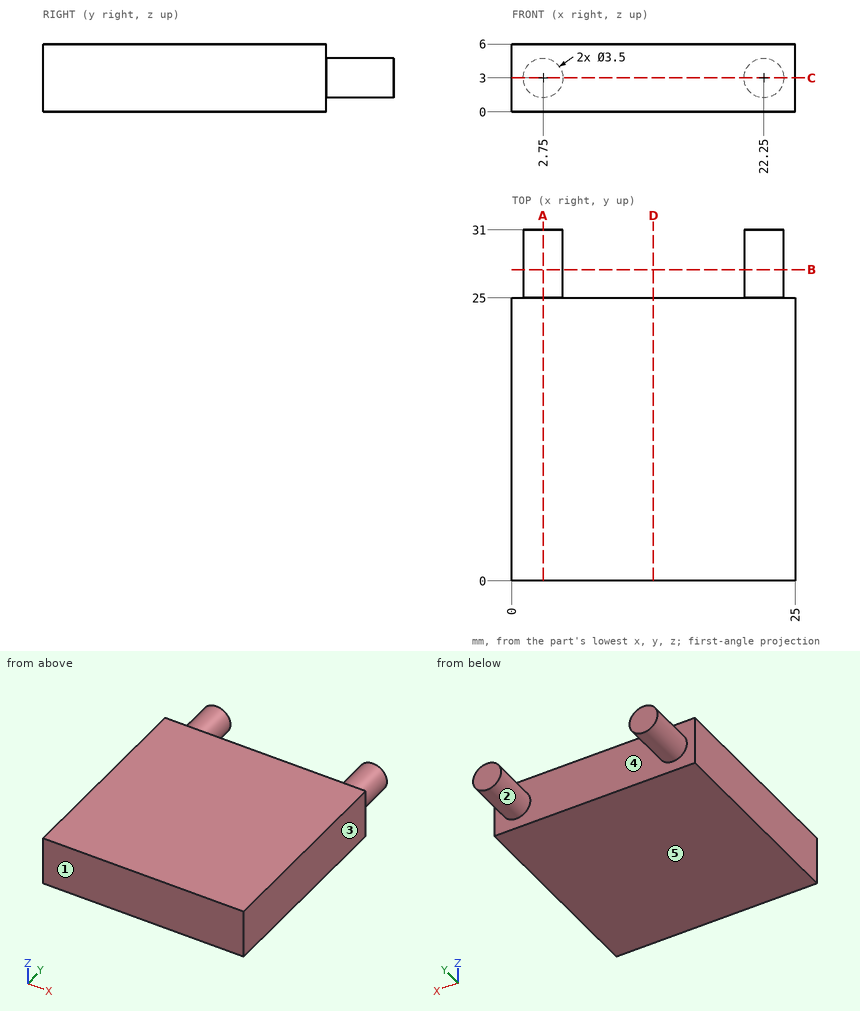
Job drawing, mm, ordinate dimensions from the low corner. One solid piece. A direction names the side the tool comes from. Give positions to 0.01 mm unless a question says otherwise; leave off trailing zeros. Order: outer loops, then holes, each group sorted by start corner. A loop starts at its lowest first (then second) coordinate and runs counter-clockwise, first axis right, second up. Notation, with made-up numbers: (50.5, -4.5) - (64.5, -4.5) arc R28 ccw to (64.5, 18.5) - close; hole circle Ø11 at (5, 78.25). An arc over 180 degrees is marked (long way). Return JSON: item names as keys, results as strings.
1) Cut at C-C, the plane z = 3. Give the cut face in (x, y).
Geometry says:
{"outline": "(0, 0) - (25, 0) - (25, 25) - (24, 25) - (24, 31) - (20.5, 31) - (20.5, 25) - (4.5, 25) - (4.5, 31) - (1, 31) - (1, 25) - (0, 25) - close"}
2) Cut at D-D, the plane x = 12.5. Give the cut face in (y, z).
Geometry says:
{"outline": "(0, 0) - (25, 0) - (25, 6) - (0, 6) - close"}
3) Cut at B-B, the plane y = 27.5. Give the cut face in (x, z), plus the area to 3 significant figures.
Geometry says:
{"outline": "circle Ø3.5 at (2.75, 3); circle Ø3.5 at (22.25, 3)", "area": "19.2 mm²"}
4) Pull direction X, two halves, no side cores. Call the marked faces 3, 4 and 5: pulls with the +X half, pulls with the -X half, needs draft (parallel to the pull), parting line crosses it, or undercut.
Geometry says:
{"face 3": "pulls with the +X half", "face 4": "undercut", "face 5": "needs draft"}
5) Cut at A-A, the plane x = 2.75. Give the cut face in (y, z).
Geometry says:
{"outline": "(0, 0) - (25, 0) - (25, 1.25) - (31, 1.25) - (31, 4.75) - (25, 4.75) - (25, 6) - (0, 6) - close"}
6) 3-axis set-ups, long thin cutter, end or side, ignore diameter. For the marked faces 1 and 2: which of +Z, -Z, +X, -X, +Y, -Y reach the whole face in a straight line?
Geometry says:
{"face 1": "+Z, -Z, +X, -X, -Y", "face 2": "+Y"}
7) Probe line 1 (Y direction, x = 8, z = 2.8). List the from-to ranges inside material, lowest first. Write a range as from..to.
Geometry says:
{"line 1": "0..25"}
